Autodesk Inventor part; units mm, degrees
ref_plane "YZ Plane" through (0, 0, 0) normal (1, 0, 0) x (0, 1, 0)
ref_plane "XZ Plane" through (0, 0, 0) normal (0, 1, 0) x (-1, 0, 0)
ref_plane "XY Plane" through (0, 0, 0) normal (0, 0, 1) x (1, 0, 0)
sketch "草圖1" plane through (0, 0, 0) normal (0, 1, 0) x (-1, 0, 0)
  line L0 (-30, 20) -> (30, 20)
  line L1 (30, 20) -> (30, -20)
  line L2 (30, -20) -> (-30, -20)
  line L3 (-30, -20) -> (-30, 20)
  line L4 (-30, 20) -> (30, -20) construction
  line L5 (30, 20) -> (-30, -20) construction
  point P0 (0, 0)
  dimension "d0" = 40
  dimension "d1" = 60
extrude "擠出1" add sketch "草圖1" along normal blind 40
sketch "草圖2" plane through (-30, 0, -20) normal (-1, 0, 0) x (0, 0, 1)
  line L0 (40, 40) -> (0, 40) construction
  line L1 (20, 40) -> (40, 20)
  line L2 (40, 20) -> (40, 40)
  line L3 (40, 40) -> (20, 40)
  point P0 (20, 0)
  dimension "d4" = 20
loft "斷面混成1" cut profiles "草圖2" section 2 point at (30, 40, 20)
sketch "草圖4" plane through (30, 0, 20) normal (1, 0, 0) x (0, 0, -1)
  line L0 (0, 40) -> (40, 40) construction
  line L1 (40, 40) -> (40, 0) construction
  line L2 (40, 0) -> (0, 0) construction
  line L3 (0, 0) -> (0, 40) construction
  line L4 (0, 20) -> (20, 40) construction
  line L5 (20, 40) -> (40, 20)
  line L6 (40, 0) -> (40, 40) construction
  line L7 (40, 20) -> (40, 40)
  line L8 (40, 40) -> (20, 40)
  line L9 (40, 40) -> (20, 40)
  point P0 (20, 0)
  dimension "d9" = 20
loft "斷面混成2" cut profiles "草圖4" section 2 point at (-30, 40, -20)
properties part number "14" material "鋼、碳鋼"
Can you work these out from the model? Positions are in its coordinate system, mm. Give positions to 0.01 mm unless a question says otherwise; leave off trailing zeros. Order: outer loops, then holes, each group sorted by start corner. A loop starts at its lowest first (then second) coordinate and runs counter-clockwise, first axis right, second up. Notation, with made-up numbers: M 82,-12 L 95,-12 A15 ccw 95,8 Z; hole C -31,-21 d9. An arc over 180 degrees is marked long. Use one line per item in the form item = value.
Item 1: Will this pin go through, and if not, where does the flat tip stop? pin 1 Ø2 at (x, y) = (22, 30) entering from -Z.
Values follow:
pin_1 = -13.72
Item 2: If we section it at D-D, the plane z = 10: Write out the boundary of the cut face in (x, y), and give its area (3 significant figures).
Values follow:
outline = M -30,0 L 30,0 L 30,40 L 0,40 L -30,30 Z
area = 2,250 mm^2
Item 3: If we section it at C-C, the plane x = -6: Write out the boundary of the cut face in (y, z).
Values follow:
outline = M 0,-20 L 32,-20 L 40,-12 L 40,8 L 28,20 L 0,20 Z
Item 4: If we section it at A-A, the plane z = -12.5: Write out the boundary of the cut face in (x, y), and give its area (3 significant figures).
Values follow:
outline = M -30,0 L 30,0 L 30,27.5 L -7.5,40 L -30,40 Z
area = 2,170 mm^2
Item 5: Thinking about a two-plate mould opening in X: for faces 1 (the flat face through (0, 15, 20)), 2 (the flat face through (30, 20, 0)), 3 (the flat face through (-30, 20, 0)), which applies, pulls with the +X half, pulls with the -X half, needs draft (parallel to the pull), parting line crosses it, or undercut?
Values follow:
face_1 = needs draft
face_2 = pulls with the +X half
face_3 = pulls with the -X half
Item 6: If we section it at B-B, the plane y = 31: Write out the boundary of the cut face in (x, z), and give its area (3 significant figures).
Values follow:
outline = M -30,-20 L -3,-20 L 30,-9 L 30,20 L 3,20 L -30,9 Z
area = 2,040 mm^2
Item 7: If I drill on line 1 along Y through (x, z) = (-3.5, 13); line 2 along Y through (x, z) = (-28, 16); line 3 along Z through (x, y) = (-3.5, 29), over which ranges is the centre line in solid material (lowest first)? Write a range as [from, to].
Values follow:
line_1 = [0, 35.83]
line_2 = [0, 24.67]
line_3 = [-20, 19.83]
